```python
from build123d import *

# Parameters (mm, degrees)
SKETCH1_R           = 0.75
SKETCH1_W           = 3.1
SKETCH1_H           = 10.1
SKETCH1_W_2         = 22
SKETCH1_H_2         = 42
SKETCH1_R_2         = 1.5
SKETCH1_W_3         = 10.1
SKETCH1_H_3         = 3.1
SKETCH1_R_3         = 9
BOSS_EXTRUDE4_DEPTH = 3
FILLET1_R           = 3


with BuildPart() as part:
    # Sketch1 → Boss-Extrude4 (new body)
    with BuildSketch(Plane.XY):
        Polygon((0, 70), (0, 0), (140, 0), (140, 120), (50, 120), (50, 70), align=None)
        with Locations((27.05, 4.5)):
            Circle(SKETCH1_R, mode=Mode.SUBTRACT)
        with Locations((4.5, 25.45)):
            Rectangle(SKETCH1_W, SKETCH1_H, mode=Mode.SUBTRACT)
        with Locations((32.05, 29.500000083)):
            Rectangle(SKETCH1_W_2, SKETCH1_H_2, mode=Mode.SUBTRACT)
        with Locations((37.05, 4.5)):
            Circle(SKETCH1_R, mode=Mode.SUBTRACT)
        with Locations((4.5, 35)):
            Circle(SKETCH1_R_2, mode=Mode.SUBTRACT)
        with Locations((4.5, 44.55)):
            Rectangle(SKETCH1_W, SKETCH1_H, mode=Mode.SUBTRACT)
        with Locations((27.05, 54.500000165)):
            Circle(SKETCH1_R, mode=Mode.SUBTRACT)
        with Locations((37.05, 54.500000165)):
            Circle(SKETCH1_R, mode=Mode.SUBTRACT)
        with Locations((102.95, 4.5)):
            Circle(SKETCH1_R, mode=Mode.SUBTRACT)
        with Locations((112.95, 4.5)):
            Circle(SKETCH1_R, mode=Mode.SUBTRACT)
        with Locations((107.95, 29.500000083)):
            Rectangle(SKETCH1_W_2, SKETCH1_H_2, mode=Mode.SUBTRACT)
        with Locations((102.95, 54.500000165)):
            Circle(SKETCH1_R, mode=Mode.SUBTRACT)
        with Locations((112.95, 54.500000165)):
            Circle(SKETCH1_R, mode=Mode.SUBTRACT)
        with Locations((135.5, 50.45)):
            Rectangle(SKETCH1_W, SKETCH1_H, mode=Mode.SUBTRACT)
        with Locations((60.45, 65.5)):
            Rectangle(SKETCH1_W_3, SKETCH1_H_3, mode=Mode.SUBTRACT)
        with Locations((70, 65.5)):
            Circle(SKETCH1_R_2, mode=Mode.SUBTRACT)
        with Locations((79.55, 65.5)):
            Rectangle(SKETCH1_W_3, SKETCH1_H_3, mode=Mode.SUBTRACT)
        with Locations((135.5, 60)):
            Circle(SKETCH1_R_2, mode=Mode.SUBTRACT)
        with Locations((135.5, 69.55)):
            Rectangle(SKETCH1_W, SKETCH1_H, mode=Mode.SUBTRACT)
        with Locations((80.128224089, 94.16)):
            Circle(SKETCH1_R_3, mode=Mode.SUBTRACT)
        with Locations((83.953224089, 115.5)):
            Rectangle(SKETCH1_W_3, SKETCH1_H_3, mode=Mode.SUBTRACT)
        with Locations((93.503224089, 115.5)):
            Circle(SKETCH1_R_2, mode=Mode.SUBTRACT)
        with Locations((103.053224089, 115.5)):
            Rectangle(SKETCH1_W_3, SKETCH1_H_3, mode=Mode.SUBTRACT)
        with Locations((106.878224089, 94.16)):
            Circle(SKETCH1_R_3, mode=Mode.SUBTRACT)
    extrude(amount=BOSS_EXTRUDE4_DEPTH)

    # Fillet1
    fillet1_edges = [part.edges().sort_by_distance(p)[0] for p in [
        (50, 120, 1.5),
        (140, 120, 1.5),
        (140, 0, 1.5),
        (0, 0, 1.5),
        (0, 70, 1.5),
        (50, 70, 1.5),
    ]]
    fillet(fillet1_edges, radius=FILLET1_R)


solid = part.part
```
Design review of the part built by this model. Coordinates are the model's own, in mm. A direction names the side the tool comes from. Give positions to 0.01 mm unless a question says otherwise; leave off trailing zeros. Order: outer loops, then holes, each group sorted by start corner. A loop starts at its lowest first (then second) coordinate and runs counter-clockwise, first axis right, second up. Notation, with made-up numbers: M -25,29.25 L 28,29.25 A25 cw 28,46.25 Z; hole C -10,48.25 d8. An arc over 180 degrees is marked long. One line per question, with ' | ' between items. Start each with the question number.
Q1. The part is to be moulded in two halves that separate along Y. For faces 1 (the face through (85, 61, 0)), 2 (the face through (25, 70, 1)), 3 (the face through (5.19, 33.67, 1.48)), say which applies: +Y half, -Y half, draft (parallel to the pull), parting line (faces both ways), or undercut.
Q2. We need section C-C (x = 135.5). Write out the cut boundary in (y, z).
Q3. For pin 1 Ø1.2 at (x, y) = (37.05, 54.5) entering from -Z; pin 2 Ø8 at (x, y) = (55, 39.5) entering from -Z; pin 3 Ø1.5 at (y, z) = (84, 1) entering from -X, all flat-tipped, find the tip position at first contact; note any pin that passes through.
Q4. We need section D-D (y = 60). Write out the cut boundary in (x, z).
Q5. For L1, parallel to X at y = 30, z = 1.6; L2, parallel to X at y = 13, z = 2.45; L3, parallel to Y at x = 135.5, z = 1.35, list the stretches that pass through material, from the lowest coordinate up. Write a range as [from, to].
Q6. Machinability: for faces 4 (the face through (103, 113.95, 1)), 5 (the face through (50.86, 119.1, 1.52)), which of the approach directions +Z, -Z, +X, -X, +Y, -Y give a long, thin tool a straight path to every point of the face, cutting with its end or side? Answer none if there is none.
Q7. We need section B-B (y = 35). Write out the cut boundary in (x, z), plus the area to 3 significant figures.
Q8. We need section A-A (x = 93.5). Write out the cut boundary in (y, z).
Returned:
1) face 1: draft | face 2: +Y half | face 3: undercut
2) outline: M 0,0 L 45.4,0 L 45.4,3 L 0,3 Z; M 55.5,0 L 58.5,0 L 58.5,3 L 55.5,3 Z; M 61.5,0 L 64.5,0 L 64.5,3 L 61.5,3 Z; M 74.6,0 L 120,0 L 120,3 L 74.6,3 Z
3) pin 1: through | pin 2: z = 0 | pin 3: x = 50
4) outline: M 0,0 L 134,0 L 134,3 L 0,3 Z; M 137,0 L 140,0 L 140,3 L 137,3 Z
5) L1: [0, 2.95], [6.05, 21.05], [43.05, 96.95], [118.95, 140] | L2: [0, 21.05], [43.05, 96.95], [118.95, 140] | L3: [0, 45.4], [55.5, 58.5], [61.5, 64.5], [74.6, 120]
6) face 4: +Z, -Z | face 5: +Z, -Z, -X, +Y
7) outline: M 0,0 L 3,0 L 3,3 L 0,3 Z; M 6,0 L 21.05,0 L 21.05,3 L 6,3 Z; M 43.05,0 L 96.95,0 L 96.95,3 L 43.05,3 Z; M 118.95,0 L 140,0 L 140,3 L 118.95,3 Z | area: 279 mm2
8) outline: M 0,0 L 114,0 L 114,3 L 0,3 Z; M 117,0 L 120,0 L 120,3 L 117,3 Z
